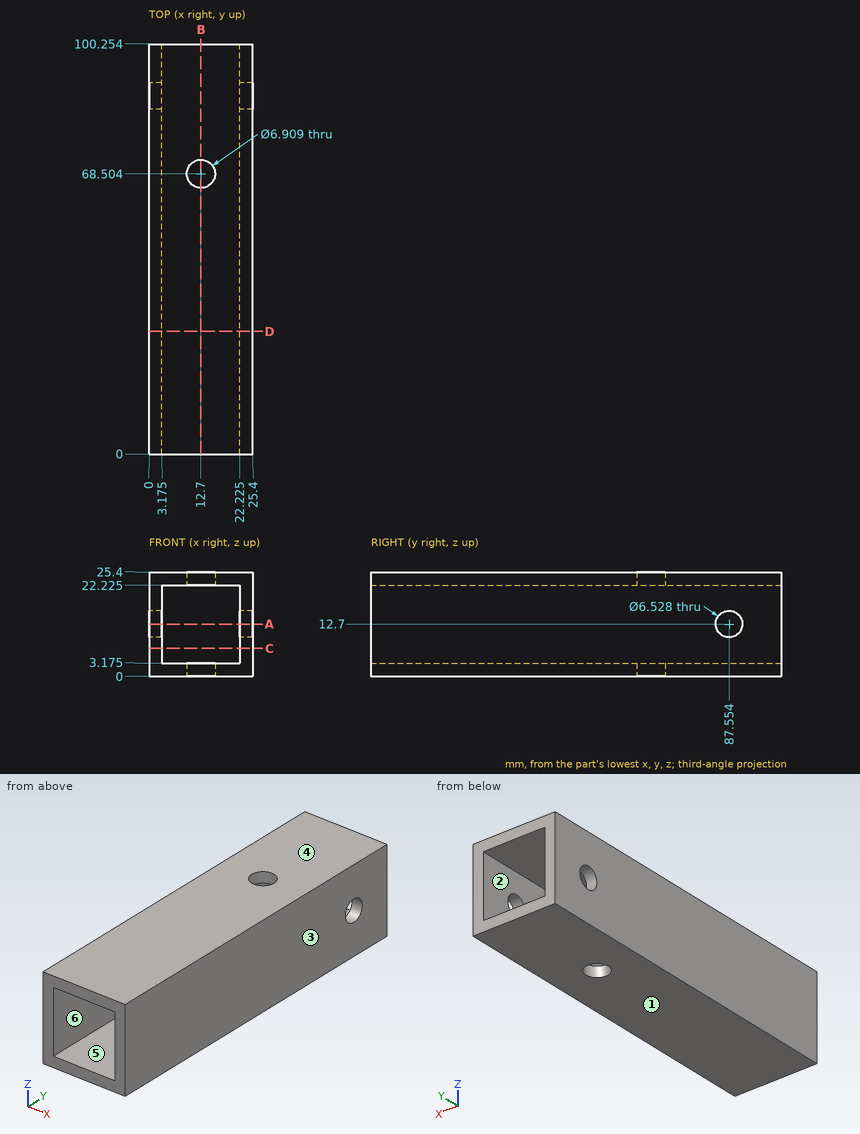
Here's the drawing with two shaded views (mm, measured from the low corner). I have some questions. A direction names the side the tool comes from. Round coordinates to 2 decimals unless told otherwise and drop trailing zeros. Loops run counter-clockwise (first coordinate to the right, second up) from the corner with the lowest first, then second, coordinate; pieces in that order, holes last. Notation, with made-up numbers: M 35.5,-17 L 82.5,-17 A21 cw 82.5,15 Z; hole C -1.5,48 d2. An arc over 180 degrees is marked long. Answer as a JSON object with one key per item and string values. Group by question number.
Q1. On a 3-axis mill with a long thin cutter (end or side, diameter ignored), from which of +Z, -Z, +X, -X, +Y, -Y can I reach the whole of each face in a straight line? I mean the marked faces 1 and 2. Say none if no direction works.
Q2. We'd pull the mould along X, two halves only. Please class the marked faces 3, 4, 5 and 6: +X half, -X half, draft (parallel to the pull), parting line (faces both ways), or undercut.
Q3. Please list where these lines run through material, in increasing order: L1, parallel to Z at x = 16.75, y = 33 (3 decimals); L2, parallel to Y at x = 12.7, z = 2.45.
Q4. Imagine slicing it at B-B, the plane x = 12.7. Please give me the cut outline in (y, z) (1 decimal).
Q5. Imagine slicing it at C-C, the plane z = 6.75. Please give me the cut outline in (x, y) (1 decimal).
Q6. Imagine slicing it at D-D, the plane y = 30. Please give me the cut outline in (x, z) (3 decimals).
Q7. Imagine slicing it at A-A, the plane z = 12.7. Please give me the cut outline in (x, y) (1 decimal), then the cut area to 3 significant figures.
Findings:
{
 "1": {"face 1": "-Z, +X, -X, +Y, -Y", "face 2": "+Y, -Y"},
 "2": {"face 3": "+X half", "face 4": "draft", "face 5": "undercut", "face 6": "undercut"},
 "3": {"L1": "z = 0 to 3.175, 22.225 to 25.4", "L2": "y = 0 to 65.05, 71.96 to 100.25"},
 "4": {"outline": "M 0,0 L 65,0 L 65,3.2 L 0,3.2 Z; M 0,22.2 L 65,22.2 L 65,25.4 L 0,25.4 Z; M 72,0 L 100.3,0 L 100.3,3.2 L 72,3.2 Z; M 72,22.2 L 100.3,22.2 L 100.3,25.4 L 72,25.4 Z"},
 "5": {"outline": "M 0,0 L 3.2,0 L 3.2,100.3 L 0,100.3 Z; M 22.2,0 L 25.4,0 L 25.4,100.3 L 22.2,100.3 Z"},
 "6": {"outline": "M 0,0 L 25.4,0 L 25.4,25.4 L 0,25.4 Z; hole M 3.175,3.175 L 22.225,3.175 L 22.225,22.225 L 3.175,22.225 Z"},
 "7": {"outline": "M 0,0 L 3.2,0 L 3.2,84.3 L 0,84.3 Z; M 0,90.8 L 3.2,90.8 L 3.2,100.3 L 0,100.3 Z; M 22.2,0 L 25.4,0 L 25.4,84.3 L 22.2,84.3 Z; M 22.2,90.8 L 25.4,90.8 L 25.4,100.3 L 22.2,100.3 Z", "area": "595 mm2"}
}
